Check sheet for the modelled part. Datum: model origin and axes. Units: mm. A direction names the side the tool comes from. Round coordinates to 2 decimals unless told otherwise and drop trailing zeros. Loops run counter-clockwise (first coordinate to the right, second up) from the corner with the lowest first, then second, coordinate; pieces in that order, holes last. Notation, with made-up numbers: M 65.5,44.25 L 103.5,44.25 A19 ccw 103.5,66.25 Z; hole C -29.75,53 d1. An arc over 180 degrees is marked long. One line per question, with ' | ' between items. Start each with the question number.
(1) Section check A-A (x = -16.75). Record the boundary of the cut face in (y, z), and give its area (3 significant figures).
(2) Draft check along X on faces 1 (the face through (-22.951, 23.253, 2.332)), 2 (the face through (-13.063, 24.23, 5.093)), 3 (the face through (-17, 26, 5.6)), 4 (the face through (-11.157, 30.149, 2.332)). Enter one of: +X half, -X half, draft (parallel to the pull), parting line (faces both ways), or undercut.
(3) Section check B-B (x = -10.5). Record the boundary of the cut face in (y, z), and give its area (3 significant figures).
(4) Section check D-D (y = 19.5). Record the boundary of the cut face in (x, z).
(5) Tool access check on faces 5 (the face through (-15, 22, 4.6)), 6 (the face through (-10.158, 23.105, 2.332)). Record the directions out of +Z, -Z, +X, -X, +Y, -Y that give a thin tool (end or side, any length) a straight path to the whole face; none if there is none.
(6) Section check C-C (z = 3.8). Count the separate pieces of the cut face and the enclosed holes in it, and give its area (3 significant figures).
(7) Thickness scan on probe 1 along Y at (x, z) = (-11, 4.05); probe 2 along Y at (x, z) = (-16, 0.7); probe 3 along X at (y, z) = (23, 4.5). Record the ranges inside material, lowest first. Write a range as [from, to].
(8) Go/stop test with flat-tipped pins: P1, Ø3, axis at x = -9.76, y = 25.76, coming from the +Z side; P2, Ø1.5, axis at x = -10, z = 3, coming from the -Y side; P3, Ø2, axis at y = 23, z = 4, coming from the +X side; P4, Ø3, axis at x = -10.7, y = 29.26, coming from the -Z side. Record where each tip stops, or that it passes through.
```python
from build123d import *

# Parameters (mm, degrees)
ESQUISSE1_R                  = 9.5
BOSS_EXTRU_1_DEPTH           = 4.6
R_P_TITION_CIRCULAIRE1_COUNT = 12
ESQUISSE2_R                  = 4
BOSS_EXTRU_4_DEPTH           = 1
ESQUISSE7_R                  = 1
ENL_V_MAT_EXTRU_1_DEPTH      = 4.6
R_P_TITION_CIRCULAIRE2_COUNT = 12


with BuildPart() as part:
    # Esquisse1 → Boss.-Extru.1 (new body)
    with BuildSketch(Plane.XY):
        with Locations((-16.758163119, 25.761769115)):
            Circle(ESQUISSE1_R)
    boss_extru_1 = extrude(amount=BOSS_EXTRU_1_DEPTH)


with BuildPart() as r_p_tition_circulaire1_1:
    # Répétition circulaire1: pattern copy
    add(boss_extru_1.rotate(Axis((-16.758163119, 25.761769115, 4.6), (0, 0, 1)), 1 * 360 / R_P_TITION_CIRCULAIRE1_COUNT))


with BuildPart() as r_p_tition_circulaire1_2:
    # Répétition circulaire1: pattern copy
    add(boss_extru_1.rotate(Axis((-16.758163119, 25.761769115, 4.6), (0, 0, 1)), 2 * 360 / R_P_TITION_CIRCULAIRE1_COUNT))


with BuildPart() as r_p_tition_circulaire1_3:
    # Répétition circulaire1: pattern copy
    add(boss_extru_1.rotate(Axis((-16.758163119, 25.761769115, 4.6), (0, 0, 1)), 3 * 360 / R_P_TITION_CIRCULAIRE1_COUNT))


with BuildPart() as r_p_tition_circulaire1_4:
    # Répétition circulaire1: pattern copy
    add(boss_extru_1.rotate(Axis((-16.758163119, 25.761769115, 4.6), (0, 0, 1)), 4 * 360 / R_P_TITION_CIRCULAIRE1_COUNT))


with BuildPart() as r_p_tition_circulaire1_5:
    # Répétition circulaire1: pattern copy
    add(boss_extru_1.rotate(Axis((-16.758163119, 25.761769115, 4.6), (0, 0, 1)), 5 * 360 / R_P_TITION_CIRCULAIRE1_COUNT))


with BuildPart() as r_p_tition_circulaire1_6:
    # Répétition circulaire1: pattern copy
    add(boss_extru_1.rotate(Axis((-16.758163119, 25.761769115, 4.6), (0, 0, 1)), 6 * 360 / R_P_TITION_CIRCULAIRE1_COUNT))


with BuildPart() as r_p_tition_circulaire1_7:
    # Répétition circulaire1: pattern copy
    add(boss_extru_1.rotate(Axis((-16.758163119, 25.761769115, 4.6), (0, 0, 1)), 7 * 360 / R_P_TITION_CIRCULAIRE1_COUNT))


with BuildPart() as r_p_tition_circulaire1_8:
    # Répétition circulaire1: pattern copy
    add(boss_extru_1.rotate(Axis((-16.758163119, 25.761769115, 4.6), (0, 0, 1)), 8 * 360 / R_P_TITION_CIRCULAIRE1_COUNT))


with BuildPart() as r_p_tition_circulaire1_9:
    # Répétition circulaire1: pattern copy
    add(boss_extru_1.rotate(Axis((-16.758163119, 25.761769115, 4.6), (0, 0, 1)), 9 * 360 / R_P_TITION_CIRCULAIRE1_COUNT))


with BuildPart() as r_p_tition_circulaire1_10:
    # Répétition circulaire1: pattern copy
    add(boss_extru_1.rotate(Axis((-16.758163119, 25.761769115, 4.6), (0, 0, 1)), 10 * 360 / R_P_TITION_CIRCULAIRE1_COUNT))


with BuildPart() as r_p_tition_circulaire1_11:
    # Répétition circulaire1: pattern copy
    add(boss_extru_1.rotate(Axis((-16.758163119, 25.761769115, 4.6), (0, 0, 1)), 11 * 360 / R_P_TITION_CIRCULAIRE1_COUNT))


with BuildPart() as part_1:
    add(part.part)

    # Répétition circulaire1 united with what: union Répétition circulaire1_1, Répétition circulaire1_2, Répétition circulaire1_3, Répétition circulaire1_4, Répétition circulaire1_5, Répétition circulaire1_6, Répétition circulaire1_7, Répétition circulaire1_8, Répétition circulaire1_9, Répétition circulaire1_10, Répétition circulaire1_11
    add(r_p_tition_circulaire1_1.part)
    add(r_p_tition_circulaire1_2.part)
    add(r_p_tition_circulaire1_3.part)
    add(r_p_tition_circulaire1_4.part)
    add(r_p_tition_circulaire1_5.part)
    add(r_p_tition_circulaire1_6.part)
    add(r_p_tition_circulaire1_7.part)
    add(r_p_tition_circulaire1_8.part)
    add(r_p_tition_circulaire1_9.part)
    add(r_p_tition_circulaire1_10.part)
    add(r_p_tition_circulaire1_11.part)

    # Esquisse2 → Boss.-Extru.4 (add)
    with BuildSketch(Plane.XY.offset(4.6)):
        with Locations((-16.758163119, 25.761769115)):
            Circle(ESQUISSE2_R)
    extrude(amount=BOSS_EXTRU_4_DEPTH)

    # Esquisse7 → Enlèv. mat.-Extru.1 (cut)
    with BuildSketch(Plane.XY.offset(4.6)):
        with Locations((-16.758163119, 32.761769115)):
            Circle(ESQUISSE7_R)
    enl_v_mat_extru_1 = extrude(amount=-ENL_V_MAT_EXTRU_1_DEPTH, mode=Mode.SUBTRACT)

    # Répétition circulaire2: Enlèv. mat.-Extru.1 ×12 about axis
    r_p_tition_circulaire2_axis = Axis((-16.758163119, 25.761769115, 0), (0, 0, 1))
    for i in range(1, R_P_TITION_CIRCULAIRE2_COUNT):
        add(enl_v_mat_extru_1.rotate(r_p_tition_circulaire2_axis, i * 360 / R_P_TITION_CIRCULAIRE2_COUNT), mode=Mode.SUBTRACT)


solid = part_1.part
```
The answers:
1) outline: M 16.26,0 L 17.76,0 L 17.76,4.6 L 16.26,4.6 Z; M 19.76,0 L 31.76,0 L 31.76,4.6 L 29.76,4.6 L 29.76,5.6 L 21.76,5.6 L 21.76,4.6 L 19.76,4.6 Z; M 33.76,0 L 35.26,0 L 35.26,4.6 L 33.76,4.6 Z | area: 77.0 mm²
2) face 1: undercut | face 2: parting line | face 3: draft | face 4: undercut
3) outline: M 18.61,0 L 21.28,0 L 21.28,4.6 L 18.61,4.6 Z; M 23.24,0 L 25.09,0 L 25.09,4.6 L 23.24,4.6 Z; M 26.43,0 L 28.28,0 L 28.28,4.6 L 26.43,4.6 Z; M 30.24,0 L 32.91,0 L 32.91,4.6 L 30.24,4.6 Z | area: 41.5 mm²
4) outline: M -23.9,0 L -21.24,0 L -21.24,4.6 L -23.9,4.6 Z; M -19.28,0 L -17.43,0 L -17.43,4.6 L -19.28,4.6 Z; M -16.08,0 L -14.24,0 L -14.24,4.6 L -16.08,4.6 Z; M -12.28,0 L -9.61,0 L -9.61,4.6 L -12.28,4.6 Z
5) face 5: +Z | face 6: +Z, -Z
6) separate pieces: 1 | enclosed holes: 12 | area: 246 mm²
7) probe 1: [18.21, 21.31], [23.21, 28.31], [30.21, 33.32] | probe 2: [16.29, 18.11], [19.41, 32.11], [33.41, 35.23] | probe 3: [-25.85, -23.49], [-22.15, -11.37], [-10.02, -7.67]
8) P1: z = 4.6 | P2: y = 18.4 | P3: x = -7.42 | P4: z = 0
